```python
from build123d import *

# Parameters (mm, degrees)
F0_W     = 120
F0_H     = 25.4
F1_DEPTH = 25.4
F2_T     = -6.35
F3_W     = 5.079999955
F3_H     = 12.7
F4_DEPTH = 6.35
F5_DEPTH = 100.94976
F6_R     = 7.62


with BuildPart() as f1:
    # F0 (on Top) → F1 (new body)
    with BuildSketch(Plane.XY):
        with Locations((60, 12.7)):
            Rectangle(F0_W, F0_H)
    extrude(amount=F1_DEPTH)

    # F2
    f2_openings = [f1.faces().sort_by_distance(p)[0] for p in [
        (120, 12.7, 12.7),
    ]]
    offset(amount=F2_T, openings=f2_openings)

    # F3 (on face) → F4 (join)
    with BuildSketch(Plane.YZ.offset(120)):
        with Locations((8.8899999775, 12.7)):
            Rectangle(F3_W, F3_H)
    extrude(amount=-F4_DEPTH)

    # F5 (add): a face of the model
    f5_faces = [f1.faces().sort_by_distance(p)[0] for p in [
        (6.35, 12.7, 12.7),
    ]]
    extrude(f5_faces, amount=F5_DEPTH)

    # F6
    f6_edges = [f1.edges().sort_by_distance(p)[0] for p in [
        (60, 25.4, 25.4),
        (60, 0, 25.4),
        (60, 0, 0),
        (60, 25.4, 0),
    ]]
    fillet(f6_edges, radius=F6_R)


solid = f1.part
```
Can you work these out from the model? Positions are in its coordinate system, mm. A direction names the side the tool comes from. Coordinates: 2 decimals unless noted, no trailing zeros. Order: outer loops, then holes, each group sorted by start corner. A loop starts at its lowest first (then second) coordinate and runs counter-clockwise, first axis right, second up.
1. For faces 1 (the face through (113.65, 9, 13)), 2 (the face through (60.84, 2.173, 23.109)), 3 (the face through (114, 19.05, 13)), which set-ups out of +Z, -Z, +X, -X, +Y, -Y let a thin tool reach every point of the face, with its end or its side?
2. If we section it at B-B (x = 80.5): Please give me the cut outline in (y, z).
3. Thinking about a two-plate mould opening in Y: for faces 4 (the face through (60.84, 23.109, 2.173)), 5 (the face through (112, 14, 19.05)), 6 (the face through (120, 10, 13)), which applies, +Y half, -Y half, draft (parallel to the pull), parting line (faces both ways), or undercut?
4. If we section it at D-D (z = 9.5): Please give me the cut outline in (x, y).
5. I need wall thicknesses on line 1 (X direction, y = 9.75, z = 16); line 2 (Z direction, x = 109, y = 16.5); line 3 (X direction, y = 19, z = 15.25). Which ranges of each line are inside material? Lowest first, please.
6. If we section it at A-A (y = 16.25): Please give me the cut outline in (x, z).
7. If we section it at C-C (y = 9.25): Please give me the cut outline in (x, z).
8. I'm going to push a flat-ended pin straight in: pin 1 (2 mm diameter, centred on y = 14.5, z = 8.5, fed in from +X). Where does the tip first touch, or does it pass through?
Entries:
1. face 1: none
1. face 2: +Z, +X, -X, -Y
1. face 3: +X
2. outline: (0, 7.62) arc R7.62 ccw to (7.62, 0) - (17.78, 0) arc R7.62 ccw to (25.4, 7.62) - (25.4, 17.78) arc R7.62 ccw to (17.78, 25.4) - (7.62, 25.4) arc R7.62 ccw to (0, 17.78) - close
3. face 4: +Y half
3. face 5: undercut
3. face 6: draft
4. outline: (0, 0) - (120, 0) - (120, 11.43) - (113.65, 11.43) - (113.65, 6.35) - (107.3, 6.35) - (107.3, 19.05) - (120, 19.05) - (120, 25.4) - (0, 25.4) - close
5. line 1: x = 0 to 107.3, 113.65 to 120
5. line 2: z = 0 to 6.35, 19.05 to 25.4
5. line 3: x = 0 to 107.3
6. outline: (0, 0) - (120, 0) - (120, 6.35) - (107.3, 6.35) - (107.3, 19.05) - (120, 19.05) - (120, 25.4) - (0, 25.4) - close
7. outline: (0, 0) - (120, 0) - (120, 25.4) - (0, 25.4) - close; hole (107.3, 6.35) - (113.65, 6.35) - (113.65, 19.05) - (107.3, 19.05) - close
8. pin 1: stops at x = 107.3
